Can you work these out from the model? Positions are in its coordinate system, mm. Give positions to 0.01 mm unless a question says otherwise; leave off trailing zeros. Order: outer loops, then holes, each group sorted by start corner. A loop starts at its lowest first (then second) coordinate and runs counter-clockwise, first axis right, second up. Notation, with made-up numbers: (11.25, 63.5) - (35.25, 63.5) arc R9 ccw to (35.25, 74.5) - close; hole circle Ø11 at (54, 60). An arc over 180 degrees is marked (long way). Answer as CSV lines item,"result".
```python
from build123d import *

# Parameters (mm, degrees)
SKETCH1_R           = 3.3782
SKETCH1_R_2         = 9.525
SKETCH1_R_3         = 4
BOSS_EXTRUDE2_DEPTH = 6.35


with BuildPart() as part:
    # Sketch1 → Boss-Extrude2 (new body)
    # profile 1 of 4: a face of its own
    with BuildSketch(Plane(origin=(0, 0, 0), x_dir=(1, 0, 0), z_dir=(0, 1, 0))):
        with BuildLine():
            ThreePointArc((-0.701449718, 27.635062977), (-8.547313496, 18.259236264), (-19.159429046, 24.329385234))
            Line((-19.159429046, 24.329385234), (-8.932978817, -3.305679122))
            ThreePointArc((-8.932978817, -3.305679122), (-7.856533502, 5.385211819), (-0.13896483, 9.523986234))
            Line((-0.13896483, 9.523986234), (-3.087221692, 17.491097626))
            ThreePointArc((-3.087221692, 17.491097626), (-2.476851738, 20.708780169), (0.652372477, 21.67521084))
            Line((0.652372477, 21.67521084), (50.178397804, 9.432220088))
            ThreePointArc((50.178397804, 9.432220088), (52.568182882, 5.966218669), (49.41646321, 3.175))
            Line((49.41646321, 3.175), (8.980256121, 3.175))
            ThreePointArc((8.980256121, 3.175), (9.387826281, 1.610696347), (9.525, 0))
            ThreePointArc((9.525, 0), (6.735192091, -6.735192091), (0, -9.525))
            Line((0, -9.525), (101.56444, -9.525))
            ThreePointArc((101.56444, -9.525), (92.109281021, 1.151344291), (103.850244371, 9.24666012))
            Line((103.850244371, 9.24666012), (-7.94064525, 36.881723073))
            ThreePointArc((-7.94064525, 36.881723073), (-2.7265193, 33.506746613), (-0.701449718, 27.635062977))
        make_face()
    # profile 2 of 4: a face of its own
    with BuildSketch(Plane(origin=(0, 0, 0), x_dir=(1, 0, 0), z_dir=(0, 1, 0))):
        with BuildLine():
            ThreePointArc((-0.13896483, 9.523986234), (-7.856533502, 5.385211819), (-8.932978817, -3.305679122))
            ThreePointArc((-8.932978817, -3.305679122), (-5.442381435, -7.817039678), (0, -9.525))
            ThreePointArc((0, -9.525), (6.735192091, -6.735192091), (9.525, 0))
            ThreePointArc((9.525, 0), (9.387826281, 1.610696347), (8.980256121, 3.175))
            Line((8.980256121, 3.175), (4.420998548, 3.175))
            ThreePointArc((4.420998548, 3.175), (2.60687144, 3.744320082), (1.443338974, 5.248106875))
            Line((1.443338974, 5.248106875), (-0.13896483, 9.523986234))
        make_face()
        with Locations(Location((0, 0, 0), (0, 0, 270))):
            Circle(SKETCH1_R, mode=Mode.SUBTRACT)
    # profile 3 of 4: a face of its own
    with BuildSketch(Plane(origin=(0, 0, 0), x_dir=(1, 0, 0), z_dir=(0, 1, 0))):
        with Locations((101.56444, 0)):
            Circle(SKETCH1_R_2)
        with Locations(Location((101.56444, 0, 0), (0, 0, 270))):
            Circle(SKETCH1_R, mode=Mode.SUBTRACT)
    # profile 4 of 4: a face of its own
    with BuildSketch(Plane(origin=(0, 0, 0), x_dir=(1, 0, 0), z_dir=(0, 1, 0))):
        with Locations((-10.226449718, 27.635062977)):
            Circle(SKETCH1_R_2)
        with Locations(Location((-10.226449718, 27.635062977, 0), (0, 0, 270))):
            Circle(SKETCH1_R_3, mode=Mode.SUBTRACT)
    extrude(amount=BOSS_EXTRUDE2_DEPTH)


solid = part.part
```
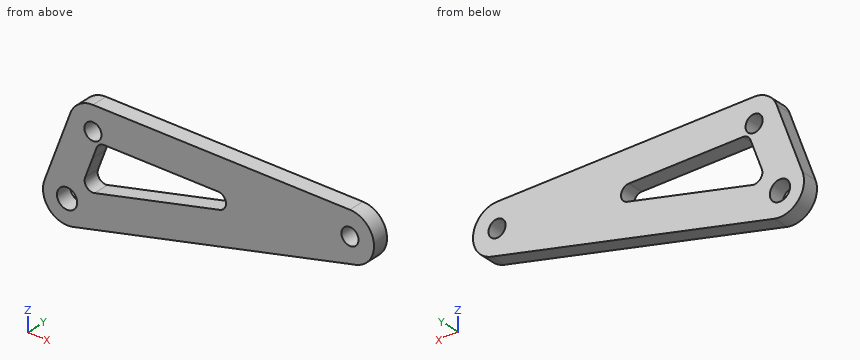
1) I want a section at A-A on z = -8. Write out the boundary of the cut face in (x, y) (3 decimals), plus the area to 3 significant figures.
Answer block:
outline,"(-13.117, 0) - (0.425, 0) - (0.425, 6.35) - (-13.117, 6.35) - close; (52.129, 0) - (106.734, 0) - (106.734, 6.35) - (52.129, 6.35) - close"
area,"433 mm2"
2) I want a section at B-B on y = 4.5. Write out the boundary of the cut face in (x, z) (3 decimals), plus the area to 3 significant figures.
Answer block:
outline,"(-19.159, -24.329) arc R9.525 ccw to (-7.941, -36.882) - (103.85, -9.247) arc R9.525 ccw to (101.564, 9.525) - (0, 9.525) arc R9.525 ccw to (-8.933, 3.306) - close; hole circle Ø8 at (-10.226, -27.635); hole circle Ø6.756 at (0, 0); hole (-3.087, -17.491) arc R3.175 ccw to (0.652, -21.675) - (50.178, -9.432) arc R3.175 ccw to (49.416, -3.175) - (4.421, -3.175) arc R3.175 ccw to (1.443, -5.248) - close; hole circle Ø6.756 at (101.564, 0)"
area,"3,260 mm2"
3) I want a section at D-D on z = 0. Write out the boundary of the cut face in (x, y).
Answer block:
outline,"(-10.16, 0) - (-3.38, 0) - (-3.38, 6.35) - (-10.16, 6.35) - close; (3.38, 0) - (98.19, 0) - (98.19, 6.35) - (3.38, 6.35) - close; (104.94, 0) - (111.09, 0) - (111.09, 6.35) - (104.94, 6.35) - close"
4) I'm going to push flat-ended pins straight in: P1, Ø1.5, axis at y = 1, z = 1.5, coming from the -X side; P2, Ø1, axis at y = 5.5, z = -1, coming from the +X side; P3, Ø6.5, axis at x = -10.23, z = -27.64, coming from the +Y side; P4, Ø1.5, axis at y = 5, z = 4, coming from the -X side. Where does each tip first touch, or does it pass through?
Answer block:
P1,"x = -9.88"
P2,"x = 111.08"
P3,"through"
P4,"x = -8.95"
5) I need wall thicknesses on line 1 along X through (y, z) = (4.5, 0); line 2 along X through (y, z) = (4.5, -0.5); line 3 along Z through (x, y) = (-8.5, 3.5). Which ranges of each line are inside material? Lowest first, please. Write a range as [from, to].
Answer block:
line 1,"[-10.16, -3.38], [3.38, 98.19], [104.94, 111.09]"
line 2,"[-10.34, -3.34], [3.34, 98.22], [104.91, 111.08]"
line 3,"[-37, -31.24], [-24.03, 4.3]"
6) I want a section at C-C on x = 17. Write out the boundary of the cut face in (y, z) (3 decimals).
Answer block:
outline,"(0, -30.716) - (6.35, -30.716) - (6.35, -17.634) - (0, -17.634) - close; (0, -3.175) - (6.35, -3.175) - (6.35, 9.525) - (0, 9.525) - close"
